Autodesk Fusion 360 part; units mm, degrees
sketch "Sketch1" plane through (0, 0, 0) normal (0, 0, 1) x (1, 0, 0)
  circle A0 centre (-35, 0) radius 6
  circle A1 centre (35, 0) radius 6
  line L0 (-39.2857, 14.3747) -> (-7.1429, 23.9579)
  line L1 (-39.2857, -14.3747) -> (-7.1429, -23.9579)
  line L2 (7.1429, 23.9579) -> (39.2857, 14.3747)
  line L3 (7.1429, -23.9579) -> (39.2857, -14.3747)
  arc A2 (39.2857, -14.3747) -> (39.2857, 14.3747) centre (35, 0) ccw
  arc A3 (-39.2857, 14.3747) -> (-39.2857, -14.3747) centre (-35, 0) ccw
  arc A4 (-7.1429, -23.9579) -> (7.1429, -23.9579) centre (0, 0) ccw
  arc A5 (7.1429, 23.9579) -> (-7.1429, 23.9579) centre (0, 0) ccw
  dimension "d3" = 50
  dimension "d4" = 12
  dimension "d5" = 12
  dimension "d6" = 35
  dimension "d7" = 35
  dimension "d8" = 30
  dimension "d9" = 30
extrude "Extrude1" add sketch "Sketch1" along normal blind 10
sketch "Sketch2" plane through (0, 0, 10) normal (0, 0, 1) x (-1, 0, 0)
  circle A0 centre (-35, 0) radius 6
  circle A1 centre (35, 0) radius 6
  arc A2 (39.2857, -14.3747) -> (39.2857, 14.3747) centre (35, 0) ccw
  line L0 (39.2857, 14.3747) -> (7.1429, 23.9579)
  arc A3 (7.1429, 23.9579) -> (-7.1429, 23.9579) centre (0, 0) ccw
  line L1 (-7.1429, 23.9579) -> (-39.2857, 14.3747)
  arc A4 (-39.2857, 14.3747) -> (-39.2857, -14.3747) centre (-35, 0) ccw
  line L2 (-39.2857, -14.3747) -> (-7.1429, -23.9579)
  arc A5 (-7.1429, -23.9579) -> (7.1429, -23.9579) centre (0, 0) ccw
  line L3 (7.1429, -23.9579) -> (39.2857, -14.3747)
  circle A6 centre (0, 0) radius 25
  circle A7 centre (0, 0) radius 15
  circle A8 centre (0, 0) radius 10
  dimension "d12" = 50
  dimension "d13" = 30
  dimension "d14" = 20
extrude "Extrude2" add sketch "Sketch2" along normal blind 28 contours A3 A5 A6
sketch "Sketch3" plane through (0, 0, 10) normal (0, 0, 1) x (-1, 0, 0)
  circle A0 centre (0, 0) radius 15
  circle A1 centre (0, 0) radius 10
  dimension "d17" = 20
extrude "Extrude3" add sketch "Sketch3" along normal blind 12
sketch "Sketch4" plane through (0, 0, 10) normal (0, 0, 1) x (-1, 0, 0)
  circle A0 centre (-35, 0) radius 6
  arc A1 (-7.1429, 23.9579) -> (-7.1429, -23.9579) centre (0, 0) ccw
  line L0 (-7.1429, 23.9579) -> (-39.2857, 14.3747)
  arc A2 (-39.2857, 14.3747) -> (-39.2857, -14.3747) centre (-35, 0) ccw
  line L1 (-39.2857, -14.3747) -> (-7.1429, -23.9579)
sketch "Sketch5" plane through (0, 0, 0) normal (1, 0, 0) x (0, 1, 0)
  circle A0 centre (0, 26) radius 3
  line L0 (25, 38) -> (-25, 38)
  dimension "d20" = 6
  dimension "d21" = 12
extrude "Extrude4" cut sketch "Sketch5" along normal blind 25
sketch "Sketch6" plane through (0, 0, 0) normal (1, 0, 0) x (0, 1, 0)
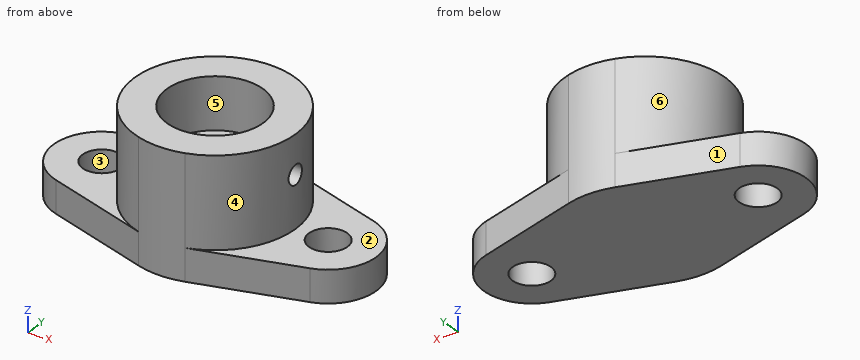
Work out the finished part from the listing and answer in its coordinate system (mm). Face numbers are marked on the shaded views. A direction names the side the tool comes from. Round coordinates to 2 decimals unless told otherwise and drop trailing zeros. Write each loop counter-clockwise with the first axis right and the second up, starting at its lowest first coordinate (ties: lowest second). Pieces come first, ordered by that corner, then holes. Notation, with made-up numbers: (7, -6) -> (41, -6) arc R13 ccw to (41, 3) -> close; hole circle Ø6 at (50, -29). An arc over 180 degrees is marked (long way). Answer as CSV lines item,"result". Start each with the question number.
(1) The part is cut by section B-B, the plane y = 0. Give the vertices of the cut face in (x, z), then the cut area to 3 significant figures.
(2) The mould has two halves that part along Y. Classify the marked faces 1, 2 and 3: +Y half, -Y half, draft (parallel to the pull), parting line (faces both ways), or undercut.
(3) Each of these flat-tipped pins is pushed along its axis until it touches: pin 1 (12 mm diameter, centred on y = -2.5, z = 28.5, fed in from +X); pin 2 (21.5 mm diameter, centred on x = -25.5, y = 10.5, fed in from +Z); pin 3 (2 mm diameter, centred on y = -13.5, z = 7, fed in from +X); pin 4 (1 mm diameter, centred on y = 13.5, z = 10, fed in from +X). Where does it stop, or does it pass through?
(4) The part is cut by section A-A, the plane z = 5. Give the vertices of the cut face in (x, y), then the cut area to 3 significant figures.
(5) A tool of negligible diameter and unlimited length cuts with its end or side. For the marked faces 4, 5 and 6, from which of +Z, -Z, +X, -X, +Y, -Y can it reach the whole face along a straight path? Write none if from no direction.
(6) The part is cut by section C-C, the plane x = 35. Give the vertices of the cut face in (y, z).
(7) The part is cut by section D-D, the plane x = 0. Give the vertices of the cut face in (y, z).
(8) Find the intervals of material crossed by probe 1 along Y at (x, z) = (-0.5, 24); probe 2 along X at (y, z) = (0, 33.5); probe 3 along Z at (x, y) = (20, 0), in increasing order.
Output values:
1,outline,"(-50, 0) -> (-41, 0) -> (-41, 10) -> (-50, 10) -> close; (-29, 0) -> (29, 0) -> (29, 10) -> (25, 10) -> (25, 23) -> (15, 23) -> (15, 22) -> (10, 22) -> (10, 10) -> (-10, 10) -> (-10, 22) -> (-15, 22) -> (-15, 38) -> (-25, 38) -> (-25, 10) -> (-29, 10) -> close; (15, 29) -> (25, 29) -> (25, 38) -> (15, 38) -> close; (41, 0) -> (50, 0) -> (50, 10) -> (41, 10) -> close"
1,area,"1,380 mm²"
2,face 1,"+Y half"
2,face 2,"draft"
2,face 3,"undercut"
3,pin 1,"stops at x = 25"
3,pin 2,"stops at z = 38"
3,pin 3,"stops at x = 43.29"
3,pin 4,"stops at x = 42.48"
4,outline,"(-39.29, -14.37) -> (-7.14, -23.96) arc R25 ccw to (7.14, -23.96) -> (39.29, -14.37) arc R15 ccw to (39.29, 14.37) -> (7.14, 23.96) arc R25 ccw to (-7.14, 23.96) -> (-39.29, 14.37) arc R15 ccw to start; hole circle Ø12 at (-35, 0); hole circle Ø12 at (35, 0)"
4,area,"3,400 mm²"
5,face 4,"+Z, +X"
5,face 5,"+Z"
5,face 6,"+Z, -X"
6,outline,"(-15.65, 0) -> (-6, 0) -> (-6, 10) -> (-15.65, 10) -> close; (6, 0) -> (15.65, 0) -> (15.65, 10) -> (6, 10) -> close"
7,outline,"(-25, 0) -> (25, 0) -> (25, 38) -> (15, 38) -> (15, 22) -> (10, 22) -> (10, 10) -> (-10, 10) -> (-10, 22) -> (-15, 22) -> (-15, 38) -> (-25, 38) -> close"
8,probe 1,"y = -25 to -14.99, 14.99 to 25"
8,probe 2,"x = -25 to -15, 15 to 25"
8,probe 3,"z = 0 to 23, 29 to 38"
